```python
from build123d import *

# Parameters (mm, degrees)
SKETCH1_R           = 2
BOSS_EXTRUDE1_DEPTH = 3
SKETCH2_R           = 1.5
CUT_EXTRUDE1_DEPTH  = 190.515777006


with BuildPart() as part:
    # Sketch1 → Boss-Extrude1 (new body)
    with BuildSketch(Plane.XY):
        with BuildLine():
            ThreePointArc((-137.970351553, -33.480224156), (-126.431132561, -39.888203569), (-124.422839539, -52.93360637))
            ThreePointArc((-124.422839539, -52.93360637), (-124.888175134, -64.31939994), (-119.594822483, -74.410646153))
            Line((-119.594822483, -74.410646153), (-92.540517723, -103.740413224))
            ThreePointArc((-92.540517723, -103.740413224), (-82.119700521, -108.557935129), (-71.344567605, -104.595807028))
            Line((-71.344567605, -104.595807028), (-37.221129556, -73.119733925))
            ThreePointArc((-37.221129556, -73.119733925), (-32.538343047, -69.892896145), (-27.140055215, -68.104192696))
            Line((-27.140055215, -68.104192696), (68.925058584, -50.795851294))
            ThreePointArc((68.925058584, -50.795851294), (82.107908339, -44.886103489), (91, -33.5))
            ThreePointArc((91, -33.5), (96.805715124, 7.17766304), (80.26119478, 44.789595257))
            ThreePointArc((80.26119478, 44.789595257), (69.434281248, 53.01522195), (56.08825014, 55.616461034))
            Line((56.08825014, 55.616461034), (-113.612396892, 49.485657177))
            ThreePointArc((-113.612396892, 49.485657177), (-129.404309407, 41.953313258), (-134.705774542, 25.279526249))
            ThreePointArc((-134.705774542, 25.279526249), (-136.343375771, 16.802270376), (-142.382746132, 10.632050724))
            ThreePointArc((-142.382746132, 10.632050724), (-155.099864059, -8.058287742), (-147.542861296, -29.364285714))
            ThreePointArc((-147.542861296, -29.364285714), (-143.125485566, -32.280163581), (-137.970351553, -33.480224156))
        make_face()
        with Locations((-81.514845762, -93.570135067)):
            Circle(SKETCH1_R, mode=Mode.SUBTRACT)
    extrude(amount=BOSS_EXTRUDE1_DEPTH)

    # Sketch2 → Cut-Extrude1 (cut, through all)
    with BuildSketch(Plane.XY.offset(3)):
        with Locations((56.196560986, 52.618416878)):
            Circle(SKETCH2_R)
        with Locations((-5.803439014, 50.378532436)):
            Circle(SKETCH2_R)
        with Locations((-67.803439014, 48.138647993)):
            Circle(SKETCH2_R)
        with Locations((68.393104802, -47.843390427)):
            Circle(SKETCH2_R)
        with Locations((7.335774003, -58.84427394)):
            Circle(SKETCH2_R)
        with Locations((-152.133709173, -14)):
            Circle(SKETCH2_R)
        with Locations((-53.721556796, -69.845157453)):
            Circle(SKETCH2_R)
    extrude(amount=-CUT_EXTRUDE1_DEPTH, mode=Mode.SUBTRACT)


solid = part.part
```
Here's how the part is built. I have some questions about the finished solid (model axes, mm). Coordinates: 2 decimals unless noted, no trailing zeros. Write each loop counter-clockwise with the first axis right and the second up, starting at its lowest first coordinate (ties: lowest second). Pieces come first, ordered by that corner, then holes. Notation, with made-up numbers: (-32.75, 53.25) - (4.25, 53.25) arc R21 ccw to (4.25, 73.25) - close; hole circle Ø10 at (1.25, -40). An arc over 180 degrees is marked (long way). One line per item, written item: value.
1) Suppose I cut it at C-C on y = 13.5. Write out the boundary of the cut face in (x, z).
Model answer:
outline: (-138.69, 0) - (95.66, 0) - (95.66, 3) - (-138.69, 3) - close
2) I need wall thicknesses on line 1 along X through (y, z) = (18.5, 2.3); line 2 along X through (y, z) = (13.5, 2.5); line 3 along Y through (x, z) = (-55, 1.25). Which ranges of each line are inside material? Lowest first, please.
Model answer:
line 1: x = -135.58 to 94.35
line 2: x = -138.69 to 95.66
line 3: y = -89.52 to -70.63, -69.06 to 51.6
3) We'd pull the mould along Y, two halves only. Please class faces 1 (the cylindrical face through (-124.923, -64.162, 1.479)), 2 (the flat face through (-31, -7, 0)), 3 (the flat face through (-54.522, -89.078, 1.479)): pulls with the +Y half, pulls with the -Y half, needs draft (parallel to the pull), parting line crosses it, or undercut.
Model answer:
face 1: undercut
face 2: needs draft
face 3: pulls with the -Y half
4) Suppose I cut it at A-A on z = 2.2. State how many separate pieces and enclosed holes the cut face has, and give its area (3 significant figures).
Model answer:
separate pieces: 1
enclosed holes: 8
area: 28,400 mm²
5) Suppose I cut it at B-B on y = -63. Write out the boundary of the cut face in (x, z), and give its area (3 significant figures).
Model answer:
outline: (-125.14, 0) - (1.19, 0) - (1.19, 3) - (-125.14, 3) - close
area: 379 mm²
